Source: three-view drawing plus pictorial views. Frame: mm from the lowest corner of the part. Round coordinates to 2 decimals unless told otherwise and drop trailing zeros. Write each loop counter-clockwise with the first axis right and the second up, starting at its lowest first coordinate (ties: lowest second). Pieces come first, ordered by that corner, then holes. Notation, with made-up numbers: (73.5, 54.25) - (95.5, 54.25) arc R15 cw to (95.5, 75.25) - close; hole circle Ø10 at (63, 82). An arc over 180 degrees is marked (long way). Write each question's results on one line, items separated by ' | '.
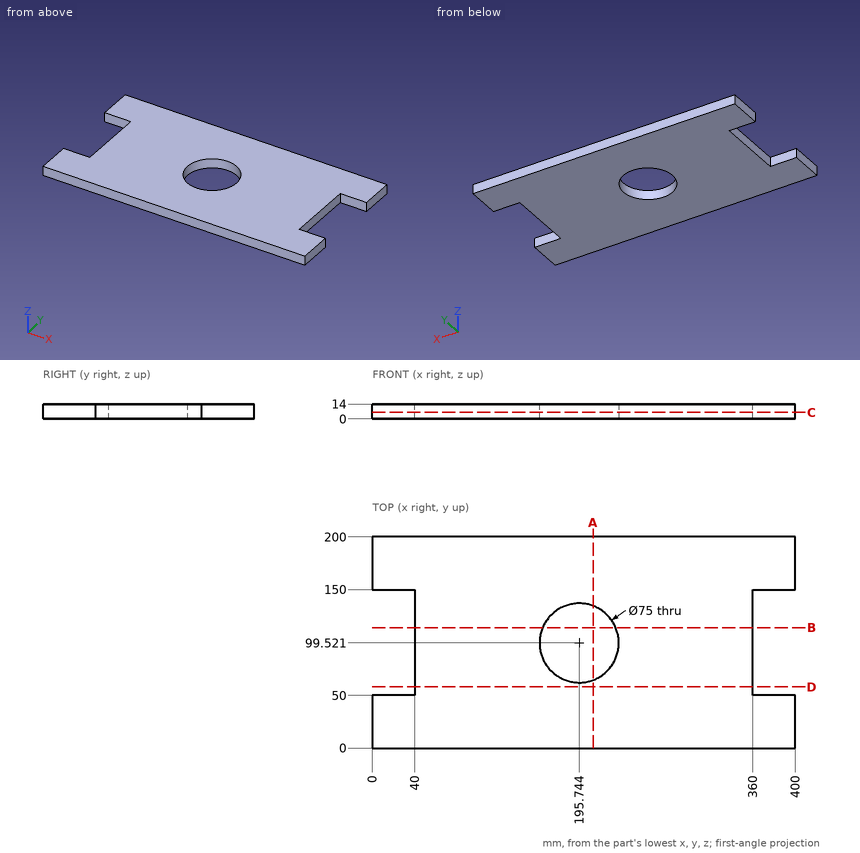
Q1. Section query D-D, the plane y = 58. Return loops of the section in (x, z), plus the area to 3 significant figures.
Answer block:
outline: (40, 0) - (360, 0) - (360, 14) - (40, 14) - close | area: 4,480 mm2
Q2. Section query A-A, the plane x = 209. Return loops of the section in (y, z).
Answer block:
outline: (0, 0) - (64.44, 0) - (64.44, 14) - (0, 14) - close; (134.6, 0) - (200, 0) - (200, 14) - (134.6, 14) - close
Q3. Section query B-B, the plane y = 114. Return loops of the section in (x, z), plus the area to 3 significant figures.
Answer block:
outline: (40, 0) - (161.15, 0) - (161.15, 14) - (40, 14) - close; (230.34, 0) - (360, 0) - (360, 14) - (230.34, 14) - close | area: 3,510 mm2
Q4. Ray query, line 1 along X through (y, z) = (100.5, 6.5); line 2 along Y through (x, z) = (37.5, 2.5); line 3 along Y through (x, z) = (164.5, 2.5) (1 decimal). Return the intervals inside material, ascending.
Answer block:
line 1: 40 to 158.26, 233.23 to 360 | line 2: 0 to 50, 150 to 200 | line 3: 0 to 78.8, 120.3 to 200
Q5. Pin query (flat end, axial travel): pin 1 (6 mm diameter, centred on y = 70.5, z = 2.5, fed in from +X); pin 2 (4 mm diameter, centred on y = 82.5, z = 3.5, fed in from -X). Return the tip coordinate at first contact, or that it passes through.
Answer block:
pin 1: x = 360 | pin 2: x = 40
Q6. Section query C-C, the plane z = 6. Return loops of the section in (x, y).
Answer block:
outline: (0, 0) - (400, 0) - (400, 50) - (360, 50) - (360, 150) - (400, 150) - (400, 200) - (0, 200) - (0, 150) - (40, 150) - (40, 50) - (0, 50) - close; hole circle Ø75 at (195.74, 99.52)
